```python
from build123d import *

# Parameters (mm, degrees)
SKETCH2_W                 = 51
SKETCH2_H                 = 12.9
BOSS_EXTRUDE1_DEPTH       = 35
M3X0_5_TAPPED_HOLE1_D     = 2.5
M3X0_5_TAPPED_HOLE1_DEPTH = 16
M3X0_5_TAPPED_HOLE1_TIP   = 0.751075774
SKETCH5_R                 = 2.2
SKETCH5_W                 = 18
SKETCH5_H                 = 5
CUT_EXTRUDE1_DEPTH        = 12.9


with BuildPart() as part:
    # Sketch2 → Boss-Extrude1 (new body)
    with BuildSketch(Plane(origin=(0, 0, 0), x_dir=(1, 0, 0), z_dir=(0, 1, 0))):
        Rectangle(SKETCH2_W, SKETCH2_H)
    extrude(amount=BOSS_EXTRUDE1_DEPTH)

    # M3x0.5 Tapped Hole1
    with Locations(Plane(origin=(0, 0, 0), x_dir=(-1, 0, 0), z_dir=(0, -1, 0))):
        with Locations((-18.75, 0), (18.75, 0)):
            Hole(M3X0_5_TAPPED_HOLE1_D / 2, depth=M3X0_5_TAPPED_HOLE1_DEPTH)
            with Locations((0, 0, -(M3X0_5_TAPPED_HOLE1_DEPTH + M3X0_5_TAPPED_HOLE1_TIP / 2))):  # 118° drill point
                Cone(0, M3X0_5_TAPPED_HOLE1_D / 2, M3X0_5_TAPPED_HOLE1_TIP, mode=Mode.SUBTRACT)

    # Sketch5 → Cut-Extrude1 (cut)
    with BuildSketch(Plane(origin=(0, 0, -6.45), x_dir=(-1, 0, 0), z_dir=(0, 0, -1))):
        with Locations((0, 20.2)):
            Circle(SKETCH5_R)
        with Locations((0, 2.5)):
            Rectangle(SKETCH5_W, SKETCH5_H)
    extrude(amount=-CUT_EXTRUDE1_DEPTH, mode=Mode.SUBTRACT)


solid = part.part
```
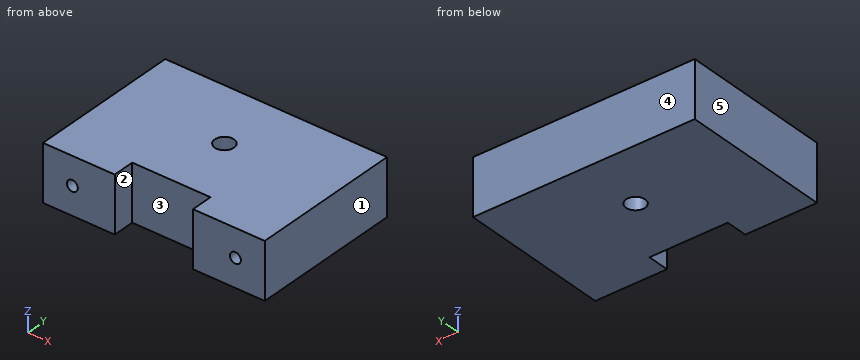
Geometry: final body of the model. Coordinates: model frame, mm. Face numbers are marked on the shaded views. A direction names the side the tool comes from. Coordinates: 2 decimals unless noted, no trailing zeros. Write each loop counter-clockwise with the first axis right and the second up, starting at its lowest first coordinate (ties: lowest second). Pieces come first, ordered by that corner, then holes. Notation, with made-up numbers: M -8.75,35 L 35.25,35 A24 ccw 35.25,59 Z; hole C -25.75,69 d9. An arc over 180 degrees is marked long. Answer as CSV lines item,"result". Start each with the question number.
Q1. Cut plane A-A on y = 2.5. Return the cut outline in (x, z), then the cut area to 3 significant figures.
Q2. Mould query, pull axis X, two halves, no side actions, for the marked faces 3, 4 and 5. Classes: released by +X, released by -X, zero draft, split by the parting line, or undercut.
Q3. Reachability of the marked faces 1 and 2 from +Z, -Z, +X, -X, +Y, -Y: full face, straight path, thin tool, end or side. Return the list, or none.
Q4. Pin query (flat end, axial travel): P1, Ø6.5, axis at x = -3.5, z = -1, coming from the -Y side; P2, Ø3.5, axis at x = 0, y = 20.2, coming from the -Z side. Return the tip coordinate at first contact, or that it passes through.
Q5. Line query: line 1 (X direction, y = 4, z = -2.5); line 2 (Y direction, x = -6, z = 6); line 3 (Y direction, x = 0, z = 0.75). Output: solid intervals per line, ascending. Write a range as from..to.
Q6. Cut plane B-B on z = 2.5. Return the cut outline in (x, y).
Q7. Cut plane D-D on y = 20.2. Return the cut outline in (x, z), then the cut area to 3 significant figures.
Q8. Cut plane C-C on x = 0. Return the cut outline in (y, z).
Findings below:
1,outline,"M -25.5,-6.45 L -9,-6.45 L -9,6.45 L -25.5,6.45 Z; M 9,-6.45 L 25.5,-6.45 L 25.5,6.45 L 9,6.45 Z; hole C -18.75,0 d2.5; hole C 18.75,0 d2.5"
1,area,"416 mm2"
2,face 3,"undercut"
2,face 4,"zero draft"
2,face 5,"released by -X"
3,face 1,"+Z, -Z, +X, +Y, -Y"
3,face 2,"+Z, -Z, -Y"
4,P1,"stops at y = 5"
4,P2,"passes through"
5,line 1,"x = -25.5..-9, 9..25.5"
5,line 2,"y = 5..35"
5,line 3,"y = 5..18, 22.4..35"
6,outline,"M -25.5,0 L -9,0 L -9,5 L 9,5 L 9,0 L 25.5,0 L 25.5,35 L -25.5,35 Z; hole C 0,20.2 d4.4"
7,outline,"M -25.5,-6.45 L -2.2,-6.45 L -2.2,6.45 L -25.5,6.45 Z; M 2.2,-6.45 L 25.5,-6.45 L 25.5,6.45 L 2.2,6.45 Z"
7,area,"601 mm2"
8,outline,"M 5,-6.45 L 18,-6.45 L 18,6.45 L 5,6.45 Z; M 22.4,-6.45 L 35,-6.45 L 35,6.45 L 22.4,6.45 Z"
